```python
from build123d import *

# Parameters (mm, degrees)
CYLINDER002_R         = 3.5
CYLINDER002_DEPTH     = 10
CYLINDER001_R         = 1.5
CYLINDER001_DEPTH     = 10
FUSION002_ROLL_ANGLE  = -90
FUSION001_PITCH_ANGLE = -90
BOX001_W              = 71
BOX001_H              = 8
BOX001_DEPTH          = 100
BOX_W                 = 103
BOX_H                 = 27
BOX_DEPTH             = 146
ARRAY_Y_COUNT         = 4
ARRAY_Y_PITCH         = 37
BOX005_W              = 43
BOX005_H              = 147
BOX005_DEPTH          = 20
BOX002_W              = 185
BOX002_H              = 175
BOX002_DEPTH          = 20


with BuildPart() as cylinder002:
    # Cylinder002 → Cylinder002 (new body)
    with BuildSketch(Plane(origin=(15, -5, 8), x_dir=(1, 0, 0), z_dir=(0, 0, 1))):
        Circle(CYLINDER002_R)
    extrude(amount=CYLINDER002_DEPTH)


with BuildPart() as cone:
    # Cone → Cone (revolve)
    with BuildSketch(Plane(origin=(15, -5, 6), x_dir=(1, 0, 0), z_dir=(0, -1, 0))):
        Polygon((0, 0), (1.5, 0), (3.5, 2), (0, 2), align=None)
    revolve(axis=Axis((15, -5, 6), (0, 0, 1)))


with BuildPart() as cylinder001:
    # Cylinder001 → Cylinder001 (new body)
    with BuildSketch(Plane(origin=(15, -5, 0), x_dir=(1, 0, 0), z_dir=(0, 0, 1))):
        Circle(CYLINDER001_R)
    extrude(amount=CYLINDER001_DEPTH)


with BuildPart() as fusion002:
    # Fusion002 base: copy of Cylinder001
    add(cylinder001.part)

    # Fusion002: union Cylinder002, Cone
    add(cylinder002.part)
    add(cone.part)


with BuildPart() as fusion002_1:
    # Fusion002 roll: moved
    add(fusion002.part.rotate(Axis((0, 0, 0), (1, 0, 0)), FUSION002_ROLL_ANGLE))


with BuildPart() as fusion002_2:
    # Fusion002 placement: moved
    add(fusion002_1.part.moved(Location((-56, -10, 5))))


with BuildPart() as fusion001:
    # Fusion001 base: copy of Cylinder001
    add(cylinder001.part)

    # Fusion001: union Cylinder002, Cone
    add(cylinder002.part)
    add(cone.part)


with BuildPart() as fusion001_1:
    # Fusion001 pitch: moved
    add(fusion001.part.rotate(Axis((0, 0, 0), (0, 1, 0)), FUSION001_PITCH_ANGLE))


with BuildPart() as fusion001_2:
    # Fusion001 placement: moved
    add(fusion001_1.part.moved(Location((113, 129.5, -5))))


with BuildPart() as cube001:
    # Box001 → Box001 (new body)
    with BuildSketch(Plane(origin=(16, 148, 0), x_dir=(1, 0, 0), z_dir=(0, 0, 1))):
        with Locations((35.5, 4)):
            Rectangle(BOX001_W, BOX001_H)
    extrude(amount=BOX001_DEPTH)


with BuildPart() as array:
    # Box → Box (new body)
    with BuildSketch(Plane.XY):
        with Locations((51.5, 13.5)):
            Rectangle(BOX_W, BOX_H)
    extrude(amount=BOX_DEPTH)

    # Array Y: Array ×4


with BuildPart() as array_1:
    add(array.part)
    with Locations(*[(0, i * ARRAY_Y_PITCH, 0) for i in range(1, ARRAY_Y_COUNT)]):
        add(array.part)


with BuildPart() as fusion:
    # Box005 → Box005 (new body)
    with BuildSketch(Plane(origin=(-62, 4, 0), x_dir=(1, 0, 0), z_dir=(0, 0, 1))):
        with Locations((21.5, 73.5)):
            Rectangle(BOX005_W, BOX005_H)
    extrude(amount=BOX005_DEPTH)

    # Fusion: union Fusion002, Fusion001, Cube001, Array
    add(fusion002_2.part)
    add(fusion001_2.part)
    add(cube001.part)
    add(array_1.part)


with BuildPart() as cut:
    # Box002 → Box002 (new body)
    with BuildSketch(Plane(origin=(-72, -10, 0), x_dir=(1, 0, 0), z_dir=(0, 0, 1))):
        with Locations((92.5, 87.5)):
            Rectangle(BOX002_W, BOX002_H)
    extrude(amount=BOX002_DEPTH)

    # Cut: cut Fusion
    add(fusion.part, mode=Mode.SUBTRACT)


solid = cut.part
```
Source: CAD feature listing. Evaluate the final solid. Frame: model axes, mm. A direction names the side the tool comes from. Give positions to 0.01 mm unless a question says otherwise; leave off trailing zeros. Write each loop counter-clockwise with the first axis right and the second up, starting at its lowest first coordinate (ties: lowest second). Pieces come first, ordered by that corner, then holes. Notation, with made-up numbers: (-39.75, 5) - (-18.75, 5) arc R18 ccw to (-18.75, 32) - close; hole circle Ø8 at (33.25, 5.5). An arc over 180 degrees is marked (long way). One line per item, written item: value. Start each with the question number.
Q1. Section query B-B, the plane y = 33. Return the cut outline in (x, z).
Q2. Draft query along Y for faces 1 (the face through (16, 152, 10)), 2 (the face through (19, -10, 10)), 3 (the face through (-72, 76, 10)). Return one class per face: +Y half, -Y half, draft (parallel to the pull), parting line (faces both ways), or undercut.
Q3. Section query A-A, the plane x = 19.5. Return the cut outline in (y, z).
Q4. Section query C-C, the plane x = 99. Return the cut outline in (y, z).
Q5. Section query D-D, the plane x = -58.5. Return the cut outline in (y, z).
Q6. Material intervals for probe 1 along X at (y, z) = (117.5, 2.25); probe 2 along Y at (x, z) = (10, 11.25); probe 3 along Y at (x, z) = (79.5, 6.75), sorted ascending. Write a range as from..to.
Q7. Set-up query: faces 4 (the face through (19, 165, 10)), 5 (the face through (104.014, 121.083, 9.241)), 6 (the face through (0, 50, 10)). Return all of +Z, -Z, +X, -X, +Y, -Y with unobstructed straight access to the full face (end or side cutting, diameter ignored); none if empty.
Answer:
1. outline: (-72, 0) - (-62, 0) - (-62, 20) - (-72, 20) - close; (-19, 0) - (113, 0) - (113, 20) - (-19, 20) - close
2. face 1: undercut
2. face 2: -Y half
2. face 3: draft
3. outline: (-10, 0) - (0, 0) - (0, 20) - (-10, 20) - close; (27, 0) - (37, 0) - (37, 20) - (27, 20) - close; (64, 0) - (74, 0) - (74, 20) - (64, 20) - close; (101, 0) - (111, 0) - (111, 20) - (101, 20) - close; (138, 0) - (148, 0) - (148, 20) - (138, 20) - close; (156, 0) - (165, 0) - (165, 20) - (156, 20) - close
4. outline: (-10, 0) - (0, 0) - (0, 20) - (-10, 20) - close; (27, 0) - (37, 0) - (37, 20) - (27, 20) - close; (64, 0) - (74, 0) - (74, 20) - (64, 20) - close; (101, 0) - (111, 0) - (111, 20) - (101, 20) - close; (138, 0) - (165, 0) - (165, 20) - (138, 20) - close
5. outline: (-10, 0) - (4, 0) - (4, 20) - (-10, 20) - close; (151, 0) - (165, 0) - (165, 20) - (151, 20) - close
6. probe 1: x = -72..-62, -19..0, 103..113
6. probe 2: y = -10..0, 27..37, 64..74, 101..111, 138..165
6. probe 3: y = -10..0, 27..37, 64..74, 101..111, 138..148, 156..165
7. face 4: +Z, -Z, +X, -X, +Y
7. face 5: none
7. face 6: +Z, -Z
